```python
from build123d import *

# Parameters (mm, degrees)
SKETCH_1_R      = 10
SKETCH_1_R_2    = 2.75
SKETCH_1_R_3    = 1.65
EXTRUDE_1_DEPTH = 5


with BuildPart() as part:
    # 草图1 → 凸台-拉伸1 (new body)
    with BuildSketch(Plane(origin=(0, 0, 0), x_dir=(-1, 0, 0), z_dir=(0, 0, -1))):
        with BuildLine():
            Line((-15, -59), (-10.25, -59))
            ThreePointArc((-10.25, -59), (-9.896446609, -58.853553391), (-9.75, -58.5))
            Line((-9.75, -58.5), (-9.75, -57.645751311))
            ThreePointArc((-9.75, -57.645751311), (-9.851137982, -57.344239966), (-10.113636364, -57.164705618))
            ThreePointArc((-10.113636364, -57.164705618), (-9.5, -52.75), (-8.886363636, -57.164705618))
            ThreePointArc((-8.886363636, -57.164705618), (-9.148862018, -57.344239966), (-9.25, -57.645751311))
            Line((-9.25, -57.645751311), (-9.25, -58.5))
            ThreePointArc((-9.25, -58.5), (-9.103553391, -58.853553391), (-8.75, -59))
            Line((-8.75, -59), (8.75, -59))
            ThreePointArc((8.75, -59), (9.103553391, -58.853553391), (9.25, -58.5))
            Line((9.25, -58.5), (9.25, -57.645751311))
            ThreePointArc((9.25, -57.645751311), (9.148862018, -57.344239966), (8.886363636, -57.164705618))
            ThreePointArc((8.886363636, -57.164705618), (9.5, -52.75), (10.113636364, -57.164705618))
            ThreePointArc((10.113636364, -57.164705618), (9.851137982, -57.344239966), (9.75, -57.645751311))
            Line((9.75, -57.645751311), (9.75, -58.5))
            ThreePointArc((9.75, -58.5), (9.896446609, -58.853553391), (10.25, -59))
            Line((10.25, -59), (15, -59))
            ThreePointArc((15, -59), (16.767766953, -58.267766953), (17.5, -56.5))
            Line((17.5, -56.5), (17.5, -50.5))
            ThreePointArc((17.5, -50.5), (17.792893219, -49.792893219), (18.5, -49.5))
            Line((18.5, -49.5), (19, -49.5))
            ThreePointArc((19, -49.5), (19.353553391, -49.353553391), (19.5, -49))
            Line((19.5, -49), (19.5, -16.332482971))
            ThreePointArc((19.5, -16.332482971), (19.604586432, -15.694198233), (19.907407407, -15.122669418))
            ThreePointArc((19.907407407, -15.122669418), (0, 25), (-19.907407407, -15.122669418))
            ThreePointArc((-19.907407407, -15.122669418), (-19.604586432, -15.694198233), (-19.5, -16.332482971))
            Line((-19.5, -16.332482971), (-19.5, -49))
            ThreePointArc((-19.5, -49), (-19.353553391, -49.353553391), (-19, -49.5))
            Line((-19, -49.5), (-18.5, -49.5))
            ThreePointArc((-18.5, -49.5), (-17.792893219, -49.792893219), (-17.5, -50.5))
            Line((-17.5, -50.5), (-17.5, -56.5))
            ThreePointArc((-17.5, -56.5), (-16.767766953, -58.267766953), (-15, -59))
        make_face()
        with Locations(Location((0, 0, 0), (0, 0, 180))):
            Circle(SKETCH_1_R, mode=Mode.SUBTRACT)
        with Locations(Location((13.856406461, 8, 0), (0, 0, 180))):
            Circle(SKETCH_1_R_2, mode=Mode.SUBTRACT)
        with Locations(Location((13.856406461, -8, 0), (0, 0, 180))):
            Circle(SKETCH_1_R_2, mode=Mode.SUBTRACT)
        with Locations(Location((0, -16, 0), (0, 0, 180))):
            Circle(SKETCH_1_R_2, mode=Mode.SUBTRACT)
        with Locations(Location((-13.856406461, -8, 0), (0, 0, 180))):
            Circle(SKETCH_1_R_2, mode=Mode.SUBTRACT)
        with Locations(Location((-13.856406461, 8, 0), (0, 0, 180))):
            Circle(SKETCH_1_R_2, mode=Mode.SUBTRACT)
        with Locations(Location((0, 16, 0), (0, 0, 180))):
            Circle(SKETCH_1_R_2, mode=Mode.SUBTRACT)
        with Locations(Location((14, -23.086792761, 0), (0, 0, 180))):
            Circle(SKETCH_1_R_3, mode=Mode.SUBTRACT)
        with Locations(Location((-14, -23.086792761, 0), (0, 0, 180))):
            Circle(SKETCH_1_R_3, mode=Mode.SUBTRACT)
        with Locations(Location((-14, -45.5, 0), (0, 0, 180))):
            Circle(SKETCH_1_R_3, mode=Mode.SUBTRACT)
        with Locations(Location((14, -45.5, 0), (0, 0, 180))):
            Circle(SKETCH_1_R_3, mode=Mode.SUBTRACT)
    extrude(amount=-EXTRUDE_1_DEPTH)


solid = part.part
```
Work out the finished part from the listing and answer in its coordinate system (mm). A direction names the side the tool comes from. Coordinates: 2 decimals unless noted, no trailing zeros. Loops run counter-clockwise (first coordinate to the right, second up) from the corner with the lowest first, then second, coordinate; pieces in that order, holes last.
1) Section A-A (y = 0) is taken. Give the vertices of the cut face in (x, z).
Results:
outline: (-25, 0) - (-10, 0) - (-10, 5) - (-25, 5) - close; (10, 0) - (25, 0) - (25, 5) - (10, 5) - close
2) For faces 4 (the flat face through (17.5, -53, 2)), 5 (the flat face through (-17.5, -54, 2)), 6 (the flat face through (-5, -16, 5)), determine the directions among +Z, -Z, +X, -X, +Y, -Y from which every point of the face is accessible in a straight line to the end or side of a thin tool.
Results:
face 4: +Z, -Z, +X, -Y
face 5: +Z, -Z, -X, -Y
face 6: +Z, +X, -X, +Y, -Y
3) Consider probe 1 along Y at (x, z) = (0, 2.45); probe 2 along X at (y, z) = (7, 4.3); probe 3 along X at (y, z) = (-6.5, 1.2). Determine where each line is inside the solid, lowest interval first.
Results:
probe 1: y = -59 to -18.75, -13.25 to -10, 10 to 13.25, 18.75 to 25
probe 2: x = -24 to -16.42, -11.29 to -7.14, 7.14 to 11.29, 16.42 to 24
probe 3: x = -24.14 to -16.16, -11.55 to -7.6, 7.6 to 11.55, 16.16 to 24.14
4) Section C-C (y = -29) is taken. Give the vertices of the cut face in (x, z), plus the area to 3 significant figures.
Results:
outline: (-19.5, 0) - (19.5, 0) - (19.5, 5) - (-19.5, 5) - close
area: 195 mm2
5) Flat-ended cylindrical pins translate along their axes: pin 1 (1.5 mm diameter, centred on y = -21.5, z = 4, fed in from -X); pin 2 (2.5 mm diameter, centred on y = -52, z = 3.5, fed in from +X); pin 3 (4.5 mm diameter, centred on x = 13.86, y = 8, fed in from -Z); pin 4 (0.7 mm diameter, centred on y = -58, z = 3, fed in from +X). Find the tip coordinate at first contact, or state that the pin passes through.
Results:
pin 1: stops at x = -19.5
pin 2: stops at x = 17.5
pin 3: passes through
pin 4: stops at x = 17.22
6) For a pull along Y with two mould halves and no side action, classify faces 1 (the cylindrical face through (-0.358, -18.727, 2.465)), 2 (the flat face through (-19.5, -33, 2)), 3 (the flat face through (0, -59, 2)) as +Y half, -Y half, draft (parallel to the pull), parting line (faces both ways), or undercut.
Results:
face 1: undercut
face 2: draft
face 3: -Y half
7) Section B-B (z = 0.8) is taken. Give the number of separate pieces and of enclosed holes in the cut face, plus the area to 3 significant figures.
Results:
separate pieces: 1
enclosed holes: 11
area: 2,840 mm2
